Model file for the job. Use its own axes, mm. Face numbers are marked on the shaded views. A direction names the side the tool comes from. Coordinates: 2 decimals unless noted, no trailing zeros. Write each loop counter-clockwise with the first axis right and the second up, starting at its lowest first coordinate (ties: lowest second). Pieces come first, ordered by that corner, then holes. Notation, with made-up numbers: M 0,58.5 L 34,58.5 A15 cw 34,66.5 Z; hole C -15.5,74 d4. An arc over 180 degrees is marked long. Answer in a Markdown table with one row per item. Add a question column.
```python
from build123d import *

# Parameters (mm, degrees)
SKETCH016_W = 1.38
SKETCH016_H = 6


with BuildPart() as part:
    # AdditivePipe005: sweep along a path in Sketch015
    with BuildLine(Plane.XY) as additivepipe005_path:
        Line((26.88, 5.5), (6.88, 5.5))
        ThreePointArc((6.88, 5.5), (2.990913, 3.889087), (1.38, 0))
        Line((1.38, 0), (1.38, -20))
    # Sketch016 → AdditivePipe005 (sweep)
    with BuildSketch(Plane.XZ):
        with Locations((0.69, 3)):
            Rectangle(SKETCH016_W, SKETCH016_H)
    sweep(path=additivepipe005_path.line)


solid = part.part
```
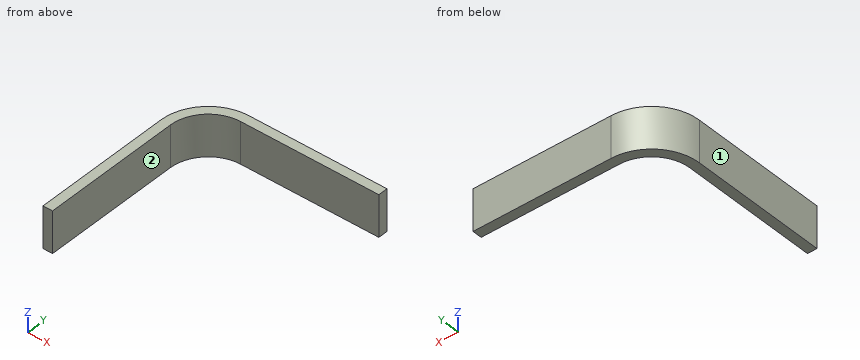
1) Slice it at C-C (y = -2). Give the cut face in (x, z), then the cut area to 3 significant figures.
2) Drill centre lines: probe 1 along Y at (x, z) = (12, 2.75); probe 2 along X at (y, z) = (-3.25, 3.5); probe 3 along X at (y, z) = (4.75, 2.25). Where is each one in solid material? Low to high.
3) Slice it at B-B (x = 16.75). Give the cut face in (y, z), then the cut area to 3 significant figures.
4) Slice it at A-A (z = 2.75). Give the cut face in (x, y), then the cut area to 3 significant figures.
5) Flat gauge pins, fed straight in: pin 1 Ø1.8 at (x, z) = (21, 3) entering from -Y; pin 2 Ø1.8 at (y, z) = (-13, 2) entering from +X. Where does each tip first touch, or does it go through?
6) Which spindle directions (+Z, -Z, +X, -X, +Y, -Y) get a long thin tool onto all of the face, cutting with end or side? Do the marked faces 1 and 2. Say none if no direction does.
Ans:
| question | item | result |
|---|---|---|
| 1 | outline | M 0,0 L 1.38,0 L 1.38,6 L 0,6 Z |
| 1 | area | 8.28 mm2 |
| 2 | probe 1 | y = 5.5 to 6.88 |
| 2 | probe 2 | x = 0 to 1.38 |
| 2 | probe 3 | x = 1.9 to 4.11 |
| 3 | outline | M 5.5,0 L 6.88,0 L 6.88,6 L 5.5,6 Z |
| 3 | area | 8.28 mm2 |
| 4 | outline | M 0,-20 L 1.38,-20 L 1.38,0 A5.5 cw 6.88,5.5 L 26.88,5.5 L 26.88,6.88 L 6.88,6.88 A6.88 ccw 0,0 Z |
| 4 | area | 68.6 mm2 |
| 5 | pin 1 | stops at y = 5.5 |
| 5 | pin 2 | stops at x = 1.38 |
| 6 | face 1 | +Z, -Z, -X, +Y, -Y |
| 6 | face 2 | +Z, -Z, +X, -Y |
